from build123d import *

# Parameters (mm, degrees)
SKETCH1_W                 = 6.042857143
SKETCH1_H                 = 5.4
SKETCH1_W_2               = 6.042857142
SKETCH1_W_3               = 4
BOSS_EXTRUDE1_DEPTH       = 3.175
BOSS_EXTRUDE2_START       = -3.175
BOSS_EXTRUDE2_OUTLINE_W   = 6.042857143
BOSS_EXTRUDE2_OUTLINE_H   = 5.4
BOSS_EXTRUDE2_OUTLINE_W_2 = 5.961577143
BOSS_EXTRUDE2_OUTLINE_H_2 = 5.31872
BOSS_EXTRUDE2_OUTLINE_W_3 = 6.042857142
BOSS_EXTRUDE2_OUTLINE_W_4 = 5.961577142
BOSS_EXTRUDE2_DEPTH       = 3.175


# Read off the part's stored shape, not the designer's step: Boss-Extrude2
with BuildPart() as part:
    # Sketch1 → Boss-Extrude1 (new body)
    # profile 1 of 4: a face of its own
    with BuildSketch(Plane.XY):
        Polygon((21.15, 38.85), (-21.15, 38.85), (-21.15, -21.15), (-13.5, -21.15), (-9.5, -21.15), (-2, -21.15), (2, -21.15), (9.5, -21.15), (13.5, -21.15), (21.15, -21.15), align=None)
        with BuildLine():
            ThreePointArc((-1.224744871, 11.25), (-1.75, 12.5), (-1.224744871, 13.75))
            ThreePointArc((-1.224744871, 13.75), (-0.67793675, 16.613351097), (1.75, 15))
            ThreePointArc((1.75, 15), (1.613351097, 14.32206325), (1.224744871, 13.75))
            ThreePointArc((1.224744871, 13.75), (1.613351097, 13.17793675), (1.75, 12.5))
            ThreePointArc((1.75, 12.5), (1.613351097, 11.82206325), (1.224744871, 11.25))
            ThreePointArc((1.224744871, 11.25), (1.613351097, 10.67793675), (1.75, 10))
            ThreePointArc((1.75, 10), (1.613351097, 9.32206325), (1.224744871, 8.75))
            ThreePointArc((1.224744871, 8.75), (1.613351097, 8.17793675), (1.75, 7.5))
            ThreePointArc((1.75, 7.5), (1.613351097, 6.82206325), (1.224744871, 6.25))
            ThreePointArc((1.224744871, 6.25), (1.613351097, 5.67793675), (1.75, 5))
            ThreePointArc((1.75, 5), (1.613351097, 4.32206325), (1.224744871, 3.75))
            ThreePointArc((1.224744871, 3.75), (1.613351097, 3.17793675), (1.75, 2.5))
            ThreePointArc((1.75, 2.5), (1.613351097, 1.82206325), (1.224744871, 1.25))
            ThreePointArc((1.224744871, 1.25), (1.613351097, 0.67793675), (1.75, 0))
            ThreePointArc((1.75, 0), (1.613351097, -0.67793675), (1.224744871, -1.25))
            ThreePointArc((1.224744871, -1.25), (1.613351097, -1.82206325), (1.75, -2.5))
            ThreePointArc((1.75, -2.5), (1.613351097, -3.17793675), (1.224744871, -3.75))
            ThreePointArc((1.224744871, -3.75), (1.613351097, -4.32206325), (1.75, -5))
            ThreePointArc((1.75, -5), (1.613351097, -5.67793675), (1.224744871, -6.25))
            ThreePointArc((1.224744871, -6.25), (1.613351097, -6.82206325), (1.75, -7.5))
            ThreePointArc((1.75, -7.5), (1.613351097, -8.17793675), (1.224744871, -8.75))
            ThreePointArc((1.224744871, -8.75), (1.613351097, -9.32206325), (1.75, -10))
            ThreePointArc((1.75, -10), (1.613351097, -10.67793675), (1.224744871, -11.25))
            ThreePointArc((1.224744871, -11.25), (1.613351097, -11.82206325), (1.75, -12.5))
            ThreePointArc((1.75, -12.5), (1.613351097, -13.17793675), (1.224744871, -13.75))
            ThreePointArc((1.224744871, -13.75), (1.613351097, -14.32206325), (1.75, -15))
            ThreePointArc((1.75, -15), (-0.67793675, -16.613351097), (-1.224744871, -13.75))
            ThreePointArc((-1.224744871, -13.75), (-1.75, -12.5), (-1.224744871, -11.25))
            ThreePointArc((-1.224744871, -11.25), (-1.75, -10), (-1.224744871, -8.75))
            ThreePointArc((-1.224744871, -8.75), (-1.75, -7.5), (-1.224744871, -6.25))
            ThreePointArc((-1.224744871, -6.25), (-1.75, -5), (-1.224744871, -3.75))
            ThreePointArc((-1.224744871, -3.75), (-1.75, -2.5), (-1.224744871, -1.25))
            ThreePointArc((-1.224744871, -1.25), (-1.75, 0), (-1.224744871, 1.25))
            ThreePointArc((-1.224744871, 1.25), (-1.75, 2.5), (-1.224744871, 3.75))
            ThreePointArc((-1.224744871, 3.75), (-1.75, 5), (-1.224744871, 6.25))
            ThreePointArc((-1.224744871, 6.25), (-1.75, 7.5), (-1.224744871, 8.75))
            ThreePointArc((-1.224744871, 8.75), (-1.75, 10), (-1.224744871, 11.25))
        make_face(mode=Mode.SUBTRACT)
        with Locations((-12.085714285, 32.65)):
            Rectangle(SKETCH1_W, SKETCH1_H, mode=Mode.SUBTRACT)
        with Locations((0, 32.65)):
            Rectangle(SKETCH1_W_2, SKETCH1_H, mode=Mode.SUBTRACT)
        with Locations((12.085714285, 32.65)):
            Rectangle(SKETCH1_W, SKETCH1_H, mode=Mode.SUBTRACT)
    # profile 2 of 4: a face of its own
    with BuildSketch(Plane.XY):
        with Locations((-11.5, -23.85)):
            Rectangle(SKETCH1_W_3, SKETCH1_H)
    # profile 3 of 4: a face of its own
    with BuildSketch(Plane.XY):
        with Locations((11.5, -23.85)):
            Rectangle(SKETCH1_W_3, SKETCH1_H)
    # profile 4 of 4: a face of its own
    with BuildSketch(Plane.XY):
        with Locations((0, -23.85)):
            Rectangle(SKETCH1_W_3, SKETCH1_H)
    extrude(amount=BOSS_EXTRUDE1_DEPTH)

    # Boss-Extrude2 outline → Boss-Extrude2 (add)
    # profile 1 of 4: a face of its own
    with BuildSketch(Plane.XY.offset(3.175).offset(BOSS_EXTRUDE2_START)):
        Polygon((13.54064, -26.59064), (13.54064, -21.19064), (21.19064, -21.19064), (21.19064, 38.89064), (-21.19064, 38.89064), (-21.19064, -21.19064), (-13.54064, -21.19064), (-13.54064, -26.59064), (-9.45936, -26.59064), (-9.45936, -21.19064), (-2.04064, -21.19064), (-2.04064, -26.59064), (2.04064, -26.59064), (2.04064, -21.19064), (9.45936, -21.19064), (9.45936, -26.59064), align=None)
        Polygon((21.15, 38.85), (21.15, -21.15), (13.5, -21.15), (13.5, -26.55), (9.5, -26.55), (9.5, -21.15), (2, -21.15), (2, -26.55), (-2, -26.55), (-2, -21.15), (-9.5, -21.15), (-9.5, -26.55), (-13.5, -26.55), (-13.5, -21.15), (-21.15, -21.15), (-21.15, 38.85), align=None, mode=Mode.SUBTRACT)
    # profile 2 of 4: a face of its own
    with BuildSketch(Plane.XY.offset(3.175).offset(BOSS_EXTRUDE2_START)):
        with Locations((12.085714285, 32.65)):
            Rectangle(BOSS_EXTRUDE2_OUTLINE_W, BOSS_EXTRUDE2_OUTLINE_H)
        with Locations((12.085714285, 32.65)):
            Rectangle(BOSS_EXTRUDE2_OUTLINE_W_2, BOSS_EXTRUDE2_OUTLINE_H_2, mode=Mode.SUBTRACT)
    # profile 3 of 4: a face of its own
    with BuildSketch(Plane.XY.offset(3.175).offset(BOSS_EXTRUDE2_START)):
        with Locations((0, 32.65)):
            Rectangle(BOSS_EXTRUDE2_OUTLINE_W_3, BOSS_EXTRUDE2_OUTLINE_H)
        with Locations((0, 32.65)):
            Rectangle(BOSS_EXTRUDE2_OUTLINE_W_4, BOSS_EXTRUDE2_OUTLINE_H_2, mode=Mode.SUBTRACT)
    # profile 4 of 4: a face of its own
    with BuildSketch(Plane.XY.offset(3.175).offset(BOSS_EXTRUDE2_START)):
        with Locations((-12.085714285, 32.65)):
            Rectangle(BOSS_EXTRUDE2_OUTLINE_W, BOSS_EXTRUDE2_OUTLINE_H)
        with Locations((-12.085714285, 32.65)):
            Rectangle(BOSS_EXTRUDE2_OUTLINE_W_2, BOSS_EXTRUDE2_OUTLINE_H_2, mode=Mode.SUBTRACT)
    extrude(amount=BOSS_EXTRUDE2_DEPTH)


solid = part.part
Can you work these out from the model? Positions are in its coordinate system, mm. A direction names the side the tool comes from. Coordinates: 2 decimals unless noted, no trailing zeros. Loops run counter-clockwise (first coordinate to the right, second up) from the corner with the lowest first, then second, coordinate; pieces in that order, holes last. Notation, with made-up numbers: (24, 10.25) - (64, 10.25) arc R11 cw to (64, 14.25) - close; hole circle Ø11 at (47.25, 9.5). An arc over 180 degrees is marked (long way). Answer as a JSON object with one key per item and string values. Group by question number.
Item 1: On a 3-axis mill with a long thin cutter (end or side, diameter ignored), from which of +Z, -Z, +X, -X, +Y, -Y can I reach the whole of each face in a straight line? I mean faces 4 (the face through (-1.75, -0.02, 1.57)), 5 (the face through (13.541, -24, 2)), 6 (the face through (-17, -21.191, 2)), 7 (the face through (-9.459, -24, 2)), 8 (the face through (-5, 7, 0)). Say none if no direction works.
Item 2: If we section it at C-C (z = 1.7): State how many separate pieces and enclosed holes the cut face has, plus the area to 3 significant figures.
Item 3: If I drill on L1, parallel to Y at x = 0, z = 1.6; L2, parallel to X at y = -23, z = 0.85; L3, parallel to X at y = -15, z = 2.5, over which ranges is the centre line in solid material (lowest first)? Write a range as from..to.
Item 4: For pin 1 (1.6 mm diameter, centred on x = -6.5, z = 1.5, fed in from -Y), with a flat end and sliding along its axis, tell me the tip position at first contact or that it passes through.
Item 5: If we section it at A-A (y = 34): List the corners of the cut face in (x, z) for me (1 decimal).
Item 6: If we mould it in two halves opening along X, with no side actions, what happens to faces 1 (the face through (21.191, 8, 2)), 2 (the face through (17, -21.191, 2)), 3 (the face through (-1.75, 4.98, 1.57))? For each: released by +X, released by -X, zero draft, split by the parting line, or undercut.
Item 7: If we section it at B-B (x = 0): List the corners of the cut face in (y, z) for me (3 decimals), plus the area to 3 significant figures.
Returned:
{
 "1": {"face 4": "+Z, -Z", "face 5": "+Z, -Z, +X, -Y", "face 6": "+Z, -Z, -X, -Y", "face 7": "+Z, -Z, -Y", "face 8": "-Z, +X, -X, +Y, -Y"},
 "2": {"separate pieces": "1", "enclosed holes": "4", "area": "2,410 mm²"},
 "3": {"L1": "y = -26.59..-16.75, 16.75..29.99, 35.31..38.89", "L2": "x = -13.54..-9.46, -2.04..2.04, 9.46..13.54", "L3": "x = -21.19..-1.75, 1.75..21.19"},
 "4": {"pin 1": "stops at y = -21.19"},
 "5": {"outline": "(-21.2, 0) - (-15.1, 0) - (-15.1, 3.2) - (-21.2, 3.2) - close; (-9.1, 0) - (-3, 0) - (-3, 3.2) - (-9.1, 3.2) - close; (3, 0) - (9.1, 0) - (9.1, 3.2) - (3, 3.2) - close; (15.1, 0) - (21.2, 0) - (21.2, 3.2) - (15.1, 3.2) - close"},
 "6": {"face 1": "released by +X", "face 2": "zero draft", "face 3": "undercut"},
 "7": {"outline": "(-26.591, 0) - (-16.75, 0) - (-16.75, 3.175) - (-26.591, 3.175) - close; (16.75, 0) - (29.991, 0) - (29.991, 3.175) - (16.75, 3.175) - close; (35.309, 0) - (38.891, 0) - (38.891, 3.175) - (35.309, 3.175) - close", "area": "84.7 mm²"}
}
